Autodesk Inventor part; units mm, degrees
ref_plane "YZ Plane" through (0, 0, 0) normal (1, 0, 0) x (0, 1, 0)
ref_plane "XZ Plane" through (0, 0, 0) normal (0, 1, 0) x (-1, 0, 0)
ref_plane "XY Plane" through (0, 0, 0) normal (0, 0, 1) x (1, 0, 0)
sketch "スケッチ1" plane through (0, 0, 0) normal (1, 0, 0) x (0, 1, 0)
  line L0 (0, 84.8101) -> (0, -115.1899)
  line L1 (0, -274.6451) -> (0, 144.7193)
  line L2 (0, 84.8101) -> (68.0158, -3.9861)
  line L3 (68.0158, -3.9861) -> (118.6619, -214.7359)
  line L4 (118.6619, -214.7359) -> (0, -115.1899)
  point P0 (0, 0)
  dimension "d0" = 200
extrude "押し出し1" add sketch "スケッチ1" along normal blind 3
chamfer "面取り1" distance 50 angle 45 1 edges at (1.5, 0, -115.1899)
fillet "フィレット1" radius 10 2 edges at (1.5, 118.6619, -214.7359) (1.5, 68.0158, -3.9861)
properties part number "type7_stay" material "CFRP"
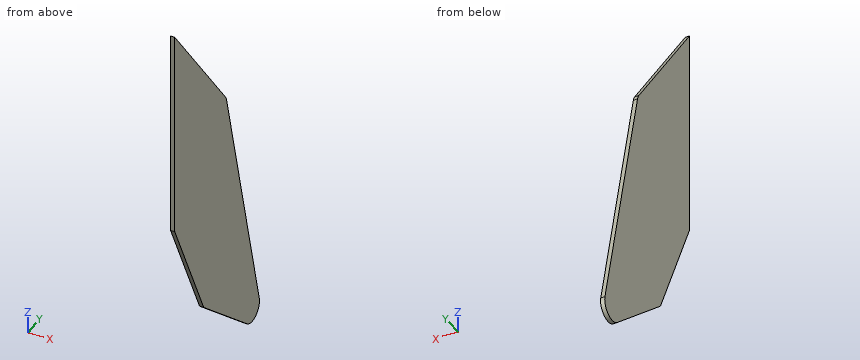
Can you work these out from the model? Positions are in its coordinate system, mm. Round coordinates to 2 decimals unless told otherwise and drop trailing zeros. Write each loop counter-clockwise with the first axis right and the second up, starting at its lowest first coordinate (ties: lowest second). Pieces come first, ordered by that corner, then holes. Notation, with made-up numbers: M 58,27 L 85,27 A16 ccw 85,55 Z; hole C 7.5,39 d5. An arc over 180 degrees is marked long. Use a Markdown table: item, result.
Item 1: I want a section at A-A (x = 2.4). List the corners of the cut face in (y, z) for me.
Found:
| item | result |
|---|---|
| outline | M 0,-65.19 L 38.31,-147.32 L 95.42,-195.24 A10 ccw 111.57,-185.24 L 68.51,-6.05 A10 ccw 66.73,-2.3 L 0,84.81 Z |
Item 2: I want a section at C-C (y = 54.5). List the corners of the cut face in (x, z) for me.
Found:
| item | result |
|---|---|
| outline | M 0,-160.91 L 3,-160.91 L 3,13.66 L 0,13.66 Z |
Item 3: I want a section at B-B (z = -129). List the corners of the cut face in (x, y) for me, and give its area (3 significant figures).
Found:
| item | result |
|---|---|
| outline | M 0,29.76 L 3,29.76 L 3,98.06 L 0,98.06 Z |
| area | 205 mm2 |
Item 4: If I drill on line 1 along Y through (x, z) = (0.4, -6); line 2 along Y through (x, z) = (0.5, -111); line 3 along Z through (x, y) = (2.4, 45.5), over which ranges is the centre line in solid material (lowest first)? Write a range as [from, to].
Found:
| item | result |
|---|---|
| line 1 | y = [0, 68.5] |
| line 2 | y = [21.36, 93.73] |
| line 3 | z = [-153.36, 25.41] |
